Autodesk Inventor part; units mm, degrees
ref_plane "YZ Plane" through (0, 0, 0) normal (1, 0, 0) x (0, 1, 0)
ref_plane "XZ Plane" through (0, 0, 0) normal (0, 1, 0) x (-1, 0, 0)
ref_plane "XY Plane" through (0, 0, 0) normal (0, 0, 1) x (1, 0, 0)
sketch "スケッチ1" plane through (0, 0, 0) normal (0, 0, 1) x (1, 0, 0)
  line L0 (0, 0) -> (15, 0)
  line L1 (15, 0) -> (15, 30)
  line L2 (15, 30) -> (0, 30)
  line L3 (0, 30) -> (0, 0)
  line L4 (1, 1) -> (14, 1)
  line L5 (14, 1) -> (14, 29)
  line L6 (14, 29) -> (1, 29)
  line L7 (1, 29) -> (1, 1)
  dimension "d0" = 15
  dimension "d1" = 30
  dimension "d2" = 13
  dimension "d3" = 28
  dimension "d4" = 1
  dimension "d5" = 1
extrude "押し出し1" add sketch "スケッチ1" along normal blind 330
sketch "スケッチ2" plane through (0, 30, 0) normal (0, 1, 0) x (1, 0, 0)
  circle A0 centre (7.5, -15) radius 1.6
  line L0 (0, 0) -> (0, -330)
  line L1 (15, 0) -> (0, 0)
  circle A1 centre (7.5, -25) radius 1.6
  circle A2 centre (7.5, -35) radius 1.6
  circle A3 centre (7.5, -315) radius 1.6
  line L2 (15, -330) -> (0, -330)
  circle A4 centre (7.5, -305) radius 1.6
  circle A5 centre (7.5, -295) radius 1.6
  dimension "d8" = 3.2
  dimension "d9" = 7.5
  dimension "d10" = 15
  dimension "d11" = 3.2
  dimension "d12" = 10
  dimension "d13" = 3.2
  dimension "d14" = 10
  dimension "d15" = 3.2
  dimension "d16" = 15
  dimension "d17" = 7.5
  dimension "d18" = 3.2
  dimension "d19" = 10
  dimension "d20" = 3.2
  dimension "d21" = 10
hole "穴1" at (7.5, 30, 315) at (7.5, 30, 305) at (7.5, 30, 295) at (7.5, 30, 15) at (7.5, 30, 25) at (7.5, 30, 35) direction (0, -1, 0) diameter 3.2 depth 30
sketch "スケッチ3" plane through (0, 0, 0) normal (-1, 0, 0) x (0, 0, 1)
  circle A0 centre (10, 15) radius 1.6
  line L0 (0, 0) -> (330, 0)
  line L1 (0, 30) -> (0, 0)
  circle A1 centre (20, 15) radius 1.6
  circle A2 centre (30, 15) radius 1.6
  circle A3 centre (320, 15) radius 1.6
  line L2 (330, 30) -> (330, 0)
  circle A4 centre (310, 15) radius 1.6
  circle A5 centre (300, 15) radius 1.6
  dimension "d29" = 3.2
  dimension "d30" = 15
  dimension "d31" = 10
  dimension "d32" = 3.2
  dimension "d33" = 3.2
  dimension "d34" = 10
  dimension "d35" = 10
  dimension "d36" = 3.2
  dimension "d37" = 15
  dimension "d38" = 10
  dimension "d39" = 3.2
  dimension "d40" = 3.2
  dimension "d41" = 10
  dimension "d42" = 10
  dimension "d43" = 15
  dimension "d44" = 15
  dimension "d45" = 15
  dimension "d46" = 15
hole "穴2" at (0, 15, 10) at (0, 15, 20) at (0, 15, 30) at (0, 15, 300) at (0, 15, 310) at (0, 15, 320) direction (1, 0, 0) diameter 3.2 depth 15
sketch "スケッチ4" plane through (0, 0, 0) normal (-1, 0, 0) x (0, 0, 1)
  line L0 (0, 22.5781) -> (0, 21.5781) construction
  line L1 (0, 1) -> (330, 1)
  line L2 (0, 22.5781) -> (1, 22.5781) construction
  line L3 (0, 30) -> (0, 0)
  dimension "d54" = 1
  dimension "d55" = 90
  dimension "d56" = 0
sketch "スケッチ5" plane through (0, 0, 0) normal (-1, 0, 0) x (0, 0, 1)
  point P0 (0, 0)
equation "\"BendRadius\" = Thickness"
equation "\"BendReliefWidth\" = Thickness"
equation "\"BendReliefDepth\" = 0.5 * Thickness"
equation "\"CornerReliefSize\" = 4 * Thickness"
equation "\"MinimumRemnant\" = 2 * Thickness"
equation "\"TransitionRadius\" = BendRadius"
equation "\"JacobiRadiusSize\" = BendRadius"
equation "\"GapSize\" = Thickness"
properties part number "nhk39"
Design review of the part built by this model. Coordinates are the model's own, in mm. A direction names the side the tool comes from. Coordinates: 2 decimals unless noted, no trailing zeros. Loops run counter-clockwise (first coordinate to the right, second up) from the corner with the lowest first, then second, coordinate; pieces in that order, holes last. Notation, with made-up numbers: (54.5, -36.75) -> (65.5, -36.75) arc R18 ccw to (65.5, -6.75) -> close; hole circle Ø2 at (86, 46). An arc over 180 degrees is marked (long way). Use a Markdown table: item, result. Add a question column.
Item 1: Machinability: for faces 4 (the flat face through (14, 15, 163)), 5 (the flat face through (0.8, 16.2, 0)), which of the approach directions +Z, -Z, +X, -X, +Y, -Y give a long, thin tool a straight path to every point of the face, cutting with its end or side? Answer none if there is none.
Item 2: We need section B-B, the plane z = 93. Write out the cut boundary in (x, y), and give its area (3 significant figures).
Item 3: We need section A-A, the plane y = 5.25. Write out the cut boundary in (x, z).
Item 4: Wall thickness on L1, parallel to X at y = 29.55, z = 295; L2, parallel to Y at x = 4.5, z = 53.5; L3, parallel to X at y = 18.5, z = 40.5: over which ranges is each line inside the solid? List them lowest first. Write a range as from..to.
Item 5: Clearance check with flat-ended pins moving along their axes: P1, Ø5, axis at y = 15, z = 10, coming from the -X side; P2, Ø1.9, axis at x = 7.5, z = 315, coming from the +Y side. State where each tip first meets the part, or that it passes through.
Item 6: The part is to be moulded in two halves that separate along Y. For faces 1 (the flat face through (7, 1, 163)), 2 (the flat face through (0.8, 16.2, 330)), 3 (the flat face through (7, 0, 163)), say which applies: +Y half, -Y half, draft (parallel to the pull), parting line (faces both ways), or undercut.
Numbers:
| question | item | result |
|---|---|---|
| 1 | face 4 | +Z, -Z |
| 1 | face 5 | -Z, +X, -X, +Y, -Y |
| 2 | outline | (0, 0) -> (15, 0) -> (15, 30) -> (0, 30) -> close; hole (1, 1) -> (14, 1) -> (14, 29) -> (1, 29) -> close |
| 2 | area | 86.0 mm^2 |
| 3 | outline | (0, 0) -> (1, 0) -> (1, 330) -> (0, 330) -> close; (14, 0) -> (15, 0) -> (15, 330) -> (14, 330) -> close |
| 4 | L1 | x = 0..5.9, 9.1..15 |
| 4 | L2 | y = 0..1, 29..30 |
| 4 | L3 | x = 0..1, 14..15 |
| 5 | P1 | stops at x = 0 |
| 5 | P2 | passes through |
| 6 | face 1 | undercut |
| 6 | face 2 | draft |
| 6 | face 3 | -Y half |
